```python
from build123d import *

# Parameters (mm, degrees)
BOSS_EXTRUDE1_DEPTH = 1
SKETCH3_W           = 2.5
SKETCH3_H           = 30
BOSS_EXTRUDE2_DEPTH = 1


with BuildPart() as part:
    # Sketch1 → Boss-Extrude1 (new body)
    with BuildSketch(Plane.XY):
        with BuildLine():
            Line((-40, 25), (40, 25))
            ThreePointArc((40, 25), (47.071067812, 22.071067812), (50, 15))
            Line((50, 15), (50, -15))
            ThreePointArc((50, -15), (47.071067812, -22.071067812), (40, -25))
            Line((40, -25), (-40, -25))
            ThreePointArc((-40, -25), (-47.071067812, -22.071067812), (-50, -15))
            Line((-50, -15), (-50, 15))
            ThreePointArc((-50, 15), (-47.071067812, 22.071067812), (-40, 25))
        make_face()
        with BuildLine():
            Line((-30, 15), (30, 15))
            ThreePointArc((30, 15), (37.071067812, 12.071067812), (40, 5))
            Line((40, 5), (40, -5))
            ThreePointArc((40, -5), (37.071067812, -12.071067812), (30, -15))
            Line((30, -15), (-30, -15))
            ThreePointArc((-30, -15), (-37.071067812, -12.071067812), (-40, -5))
            Line((-40, -5), (-40, 5))
            ThreePointArc((-40, 5), (-37.071067812, 12.071067812), (-30, 15))
        make_face(mode=Mode.SUBTRACT)
    extrude(amount=BOSS_EXTRUDE1_DEPTH)

    # Sketch3 → Boss-Extrude2 (add)
    with BuildSketch(Plane.XY.offset(1)):
        with Locations((-33.75, 0)):
            Rectangle(SKETCH3_W, SKETCH3_H)
        with Locations((-26.25, 0)):
            Rectangle(SKETCH3_W, SKETCH3_H)
        with Locations((-18.75, 0)):
            Rectangle(SKETCH3_W, SKETCH3_H)
        with Locations((-11.25, 0)):
            Rectangle(SKETCH3_W, SKETCH3_H)
        with Locations((-3.75, 0)):
            Rectangle(SKETCH3_W, SKETCH3_H)
        with Locations((3.75, 0)):
            Rectangle(SKETCH3_W, SKETCH3_H)
        with Locations((11.25, 0)):
            Rectangle(SKETCH3_W, SKETCH3_H)
        with Locations((18.75, 0)):
            Rectangle(SKETCH3_W, SKETCH3_H)
        with Locations((26.25, 0)):
            Rectangle(SKETCH3_W, SKETCH3_H)
        with Locations((33.75, 0)):
            Rectangle(SKETCH3_W, SKETCH3_H)
    extrude(amount=-BOSS_EXTRUDE2_DEPTH)


solid = part.part
```
Source: CAD feature listing. Evaluate the final solid. Frame: model axes, mm. Coordinates: 2 decimals unless noted, no trailing zeros. Return JSON: item names as keys, results as strings. Group by question number.
1) Ray query, line 1 along Y through (x, z) = (-17, 0.15); line 2 along Y through (x, z) = (32, 0.95); line 3 along X through (y, z) = (-15.5, 0.7). Return the intervals inside material, ascending.
2) Section query A-A, the plane z = 0.5. State how many separate pieces and enclosed holes the cut face has, plus the area to 3 significant figures.
3) Mould query, pull axis X, two halves, no side actions, for faces 1 (the face through (-38.697, 9.936, 0.493)), 2 (the face through (-46.99, -22.15, 0.49)), 3 (the face through (47.15, -21.99, 0.49)), 4 (the face through (38.6, 10.1, 0.5)). Classes: +X half, -X half, draft (parallel to the pull), parting line (faces both ways), or undercut.
From the geometry:
{
 "1": {"line 1": "-25 to -15, 15 to 25", "line 2": "-25 to -14.8, 14.8 to 25", "line 3": "-49.99 to 49.99"},
 "2": {"separate pieces": "1", "enclosed holes": "11", "area": "3,340 mm²"},
 "3": {"face 1": "undercut", "face 2": "-X half", "face 3": "+X half", "face 4": "undercut"}
}
